Design review of the part shown in the three views and the two pictorial views. Dimensions are in mm from the part's minimum x, y and z. Give positions to 0.01 mm unless a question says otherwise; leave off trailing zeros. Loops run counter-clockwise (first coordinate to the right, second up) from the corner with the lowest first, then second, coordinate; pieces in that order, holes last. Notation, with made-up numbers: (39, -39.75) -> (81, -39.75) arc R19 ccw to (81, -4.75) -> close; hole circle Ø1 at (53.5, 20). An arc over 180 degrees is marked (long way). Answer as CSV lines item,"result". Start each with the question number.
Item 1: Add section D-D on z = 7.25. State the section outline as (x, y) points.
Item 2: Clearance check with flat-ended pins moving along their axes: P1, Ø3, axis at x = 13, z = 5.5, coming from the -Y side; P2, Ø4, axis at y = 10, z = 11, coming from the +X side; P3, Ø3, axis at y = 15, z = 9.5, coming from the -X side; P4, Ø4, axis at x = 14.5, z = 7.5, coming from the -Y side. State where each tip first meets the part, or that it passes through.
Item 3: For L1, parallel to Y at x = 11, z = 4; L2, parallel to Y at x = 15.25, z = 8 (1 decimal), list the stretches that pass through material, from the lowest coordinate up. Write a range as from..to.
Item 4: Add section C-C on z = 1.25. State the section outline as (x, y) points.
Item 5: Add section A-A on x = 11. State the section outline as (y, z) points.
Item 6: The part is to be moulded in two halves that separate along X. For the marked faces 1, 2 and 3, say which applies: +X half, -X half, draft (parallel to the pull), parting line (faces both ways), or undercut.
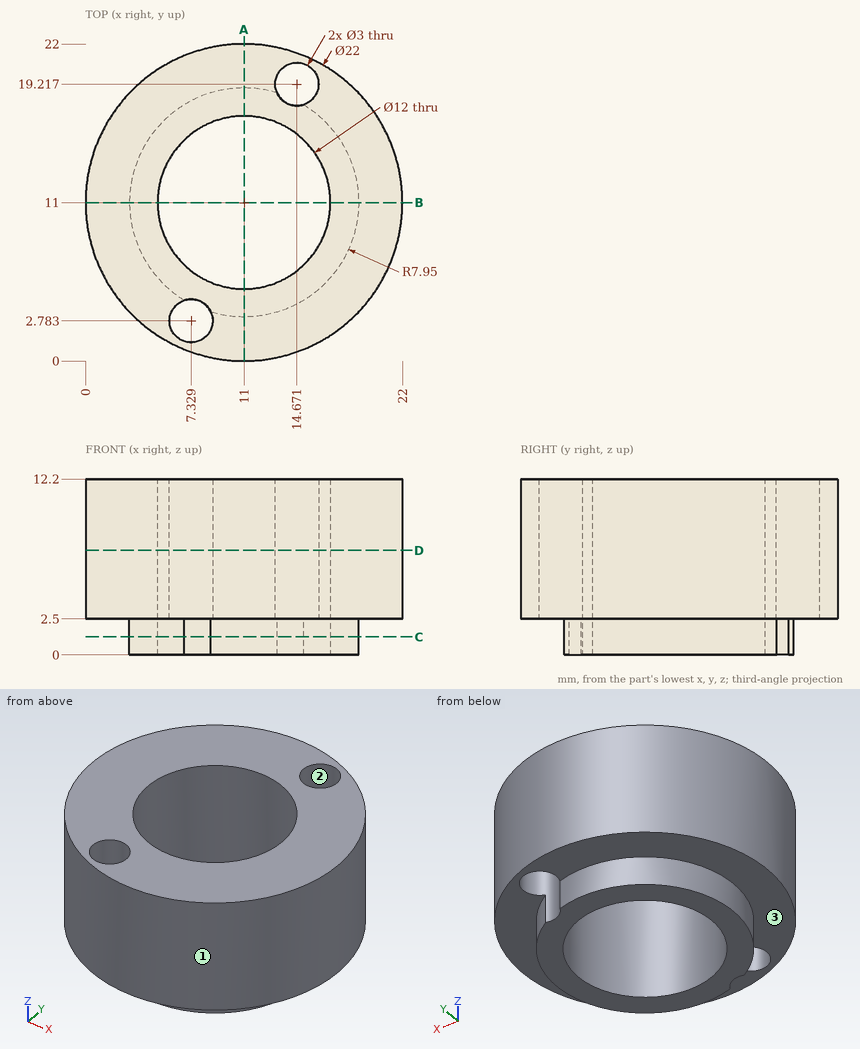
Computed values:
1,outline,"circle Ø22 at (11, 11); hole circle Ø12 at (11, 11); hole circle Ø3 at (7.33, 2.78); hole circle Ø3 at (14.67, 19.22)"
2,P1,"y = 0.01"
2,P2,"x = 22"
2,P3,"x = 0.29"
2,P4,"y = 0.1"
3,L1,"0..5, 17..22"
3,L2,"0.9..6.8, 15.2..17.8, 20.6..21.1"
4,outline,"(6.87, 4.21) arc R1.5 cw to (8.7, 3.39) arc R7.95 ccw to (15.13, 17.79) arc R1.5 cw to (13.3, 18.61) arc R7.95 ccw to start; hole circle Ø12 at (11, 11)"
5,outline,"(0, 2.5) -> (3.05, 2.5) -> (3.05, 0) -> (5, 0) -> (5, 12.2) -> (0, 12.2) -> close; (17, 0) -> (18.95, 0) -> (18.95, 2.5) -> (22, 2.5) -> (22, 12.2) -> (17, 12.2) -> close"
6,face 1,"parting line"
6,face 2,"undercut"
6,face 3,"draft"
